from build123d import *

# Parameters (mm, degrees)
ESQUISSE1_R             = 16.1
BOSS_EXTRU_1_DEPTH      = 100.3
ESQUISSE2_W             = 10
ESQUISSE2_H             = 5
ENL_V_MAT_EXTRU_1_DEPTH = 10
ENL_V_MAT_EXTRU_2_DEPTH = 10


with BuildPart() as part:
    # Esquisse1 → Boss.-Extru.1 (new body)
    with BuildSketch(Plane(origin=(0, 0, 0), x_dir=(0, 0, -1), z_dir=(1, 0, 0))):
        Circle(ESQUISSE1_R)
    extrude(amount=BOSS_EXTRU_1_DEPTH)

    # Esquisse2 → Enlèv. mat.-Extru.1 (cut)
    with BuildSketch(Plane.ZY):
        with Locations((-4, 0.220705936)):
            Rectangle(ESQUISSE2_W, ESQUISSE2_H)
    extrude(amount=-ENL_V_MAT_EXTRU_1_DEPTH, mode=Mode.SUBTRACT)

    # Esquisse3 → Enlèv. mat.-Extru.2 (cut)
    with BuildSketch(Plane.ZY):
        with BuildLine():
            Line((3.990495341, -1.5), (11.990495341, -1.5))
            ThreePointArc((11.990495341, -1.5), (11.301155513, -0.335786438), (9.990495341, 0))
            Line((9.990495341, 0), (5.990495341, 0))
            ThreePointArc((5.990495341, 0), (4.679835169, -0.335786438), (3.990495341, -1.5))
        make_face()
    extrude(amount=-ENL_V_MAT_EXTRU_2_DEPTH, mode=Mode.SUBTRACT)


solid = part.part
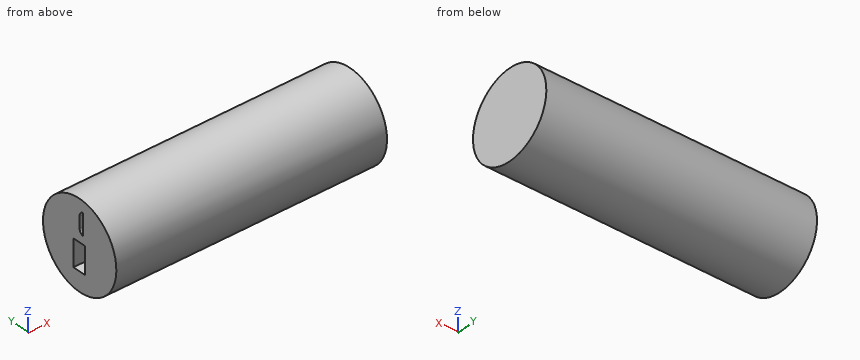
Source: CAD feature listing. Evaluate the final solid. Frame: model axes, mm. Coordinates: 2 decimals unless noted, no trailing zeros. Order: outer loops, then holes, each group sorted by start corner. A loop starts at its lowest first (then second) coordinate and runs counter-clockwise, first axis right, second up.
Item 1: Cut plane D-D (y = 10). Return loops of the section in (x, z), plus the area to 3 significant figures.
Output values:
outline: (0, -12.62) - (100.3, -12.62) - (100.3, 12.62) - (0, 12.62) - close
area: 2,530 mm2
Item 2: Cut plane A-A (z = 0). Return loops of the section in (x, y), plus the area to 3 significant figures.
Output values:
outline: (0, -16.1) - (100.3, -16.1) - (100.3, 16.1) - (0, 16.1) - (0, 2.72) - (10, 2.72) - (10, -2.28) - (0, -2.28) - close
area: 3,180 mm2
Item 3: Cut plane C-C (z = -7.5). Return loops of the section in (x, y).
Output values:
outline: (0, -14.25) - (100.3, -14.25) - (100.3, 14.25) - (0, 14.25) - (0, 2.72) - (10, 2.72) - (10, -2.28) - (0, -2.28) - close
Item 4: Cut plane B-B (x = 88.5). Return loops of the section in (y, z), plus the area to 3 significant figures.
Output values:
outline: circle Ø32.2 at (0, 0)
area: 814 mm2
Item 5: Material intervals for line 1 (X direction, y = 0.5, z = -3); line 2 (Y direction, x = 4, z = 9); line 3 (Z direction, x = 87, y = 0.5), sorted ascending.
Output values:
line 1: x = 10 to 100.3
line 2: y = -13.35 to -1.5, 0 to 13.35
line 3: z = -16.09 to 16.09
Item 6: First-contact query: P1, Ø1.5, axis at x = 3, y = -0.5, coming from the -Z side; P2, Ø1.5, axis at x = 37.5, y = -2.5, coming from the +Z side; P3, Ø12, axis at x = 16, y = -9, coming from the +Z side; P4, Ø2, axis at x = 7, z = 8, coming from the -Y side. Flat tips, straight axial feed; report the tip coordinate or a pass-through.
Output values:
P1: stops at z = -16.1
P2: stops at z = 16
P3: stops at z = 15.82
P4: stops at y = -14.5
